Part model, mm, in its own coordinate system. Round coordinates to 2 decimals unless told otherwise and drop trailing zeros. Order: outer loops, then holes, each group sorted by start corner. A loop starts at its lowest first (then second) coordinate and runs counter-clockwise, first axis right, second up. Notation, with made-up numbers: (17.25, -32.5) - (39.25, -32.5) arc R18 ccw to (39.25, -13.5) - close; hole circle Ø11 at (-8, 45.5). An arc over 180 degrees is marked (long way). Answer as a JSON object with one key per item and string values.
Autodesk Inventor part; units mm, degrees
ref_plane "YZ Plane" through (0, 0, 0) normal (1, 0, 0) x (0, 1, 0)
ref_plane "XZ Plane" through (0, 0, 0) normal (0, 1, 0) x (-1, 0, 0)
ref_plane "XY Plane" through (0, 0, 0) normal (0, 0, 1) x (1, 0, 0)
sketch "스케치1" plane through (0, 0, 0) normal (0, 0, 1) x (1, 0, 0)
  line L0 (0, 20) -> (0, 20)
  line L1 (20, 0) -> (20, 0)
  line L2 (0, -20) -> (0, -20)
  line L3 (-20, 0) -> (-20, 0)
  line L4 (0, 18) -> (0, 18)
  line L5 (-18, 0) -> (-18, 0)
  line L6 (0, -18) -> (0, -18)
  line L7 (18, 0) -> (18, 0)
  arc A0 (0, 18) -> (-18, 0) centre (0, 0) ccw
  arc A1 (-18, 0) -> (0, -18) centre (0, 0) ccw
  arc A2 (0, -18) -> (18, 0) centre (0, 0) ccw
  arc A3 (18, 0) -> (0, 18) centre (0, 0) ccw
  arc A4 (0, 20) -> (-20, 0) centre (0, 0) ccw
  arc A5 (-20, 0) -> (0, -20) centre (0, 0) ccw
  arc A6 (0, -20) -> (20, 0) centre (0, 0) ccw
  arc A7 (20, 0) -> (0, 20) centre (0, 0) ccw
  point P0 (0, 0)
  point P1 (-20, 20)
  point P2 (20, -20)
  point P3 (20, 20)
  point P4 (-20, -20)
  point P5 (18, 18)
  point P6 (-18, 18)
  point P7 (-18, -18)
  point P8 (18, -18)
  dimension "d0" = 40
  dimension "d1" = 40
  dimension "d2" = 20
  dimension "d3" = 20
  dimension "d4" = 2
  dimension "d7" = 18
  dimension "d8" = 18
  dimension "d9" = 18
  dimension "d10" = 18
  dimension "d11" = 20
extrude "돌출1" add sketch "스케치1" along normal blind 200
properties part number "링크2_240mm" material "CFRP"
Item 1: Cut at C-C (z = 43.5). Write the cut outline in (x, y).
Taken from the geometry:
{"outline": "circle Ø40 at (0, 0); hole circle Ø36 at (0, 0)"}
Item 2: Cut at A-A (y = 0). Write the cut outline in (x, z), plus the area to 3 significant figures.
Taken from the geometry:
{"outline": "(-20, 0) - (-18, 0) - (-18, 200) - (-20, 200) - close; (18, 0) - (20, 0) - (20, 200) - (18, 200) - close", "area": "800 mm2"}
Item 3: Two-plate mould, pull along Y, no slides. Class faces 1 (the flat face through (-18, 3, 200)), 2 (the cylindrical face through (-4.336, 19.524, 98.6)), 3 (the cylindrical face through (17.847, -2.343, 98.6)): pulls with the +Y half, pulls with the -Y half, needs draft (parallel to the pull), parting line crosses it, or undercut.
Taken from the geometry:
{"face 1": "needs draft", "face 2": "parting line crosses it", "face 3": "undercut"}
Item 4: Drop flat-ended pins along their axis: P1, Ø1.5, axis at x = 12, z = 43, coming from the -Y side; P2, Ø6, axis at x = -6.5, z = 162, coming from the -Y side; P3, Ø1.5, axis at x = -13.5, z = 28.5, coming from the +Y side. Give the stop position or say it passes through.
Taken from the geometry:
{"P1": "y = -16.54", "P2": "y = -19.69", "P3": "y = 15.41"}
Item 5: Probe L1, parallel to Y at x = 0, z = 128.5; L2, parallel to X at y = -9, z = 136. List the from-to ranges inside material, lowest first. Write a range as from..to.
Taken from the geometry:
{"L1": "-20..-18, 18..20", "L2": "-17.86..-15.59, 15.59..17.86"}
